Design review of the part built by this model. Coordinates are the model's own, in mm. Face numbers are marked on the shaded views. A direction names the side the tool comes from. Coordinates: 2 decimals unless noted, no trailing zeros. Loops run counter-clockwise (first coordinate to the right, second up) from the corner with the lowest first, then second, coordinate; pieces in that order, holes last.
Q1. Machinability: for the marked faces 1 and 2, which of the approach directions +Z, -Z, +X, -X, +Y, -Y give a long, thin tool a straight path to every point of the face, cutting with its end or side? Answer none if there is none.
Q2. For P1, Ø3, axis at x = 15, y = 4, coming from the -Z side; P2, Ø1, axis at x = -8.5, y = 2, coming from the +Z side; P3, Ø2, axis at x = 16, y = 3, coming from the -Z side, all flat-tipped, find the tip position at first contact; note any pin that passes through.
Q3. Add section C-C on y = 0.85. Give the boundary of the cut face in (x, z).
Q4. Add section D-D on x = 0. Give the boundary of the cut face in (y, z), and give its area (3 significant figures).
Q5. Add section A-A on x = -22. Give the boundary of the cut face in (y, z), and give its area (3 significant figures).
Q6. Draft analysis for pull direction X (two halves, no side actions). For the marked faces 3 and 4, state which applies: released by +X, released by -X, zero draft, split by the parting line, or undercut.
Q7. Add section B-B on z = -22. Give the boundary of the cut face in (x, y).
Q8. Wall thickness on probe 1 along X at (y, z) = (0.9, 1); probe 2 along X at (y, z) = (1.9, 22): over which ranges is each line inside the solid? List them lowest first.
```python
from build123d import *

# Parameters (mm, degrees)
SKETCH1_R           = 1.5
BOSS_EXTRUDE1_DEPTH = 3
BOSS_EXTRUDE2_START = 3
SKETCH1_4_R         = 1.5
SKETCH1_4_R_2       = 16
SKETCH1_4_R_3       = 13
BOSS_EXTRUDE2_DEPTH = 2


with BuildPart() as part:
    # Sketch1 → Boss-Extrude1 (new body)
    with BuildSketch(Plane(origin=(0, 0, 0), x_dir=(1, 0, 0), z_dir=(0, 1, 0))):
        with BuildLine():
            ThreePointArc((19.8125, 2.732186624), (14.142135624, 14.142135624), (2.732186624, 19.8125))
            ThreePointArc((2.732186624, 19.8125), (0, 25.5), (-2.732186624, 19.8125))
            ThreePointArc((-2.732186624, 19.8125), (-14.142135624, 14.142135624), (-19.8125, 2.732186624))
            ThreePointArc((-19.8125, 2.732186624), (-25.5, 0), (-19.8125, -2.732186624))
            ThreePointArc((-19.8125, -2.732186624), (-14.142135624, -14.142135624), (-2.732186624, -19.8125))
            ThreePointArc((-2.732186624, -19.8125), (0, -25.5), (2.732186624, -19.8125))
            ThreePointArc((2.732186624, -19.8125), (14.142135624, -14.142135624), (19.8125, -2.732186624))
            ThreePointArc((19.8125, -2.732186624), (25.5, 0), (19.8125, 2.732186624))
        make_face()
        with Locations((22, 0)):
            Circle(SKETCH1_R, mode=Mode.SUBTRACT)
        with Locations((0, 22)):
            Circle(SKETCH1_R, mode=Mode.SUBTRACT)
        with Locations((0, -22)):
            Circle(SKETCH1_R, mode=Mode.SUBTRACT)
        with Locations((-22, 0)):
            Circle(SKETCH1_R, mode=Mode.SUBTRACT)
    extrude(amount=BOSS_EXTRUDE1_DEPTH)

    # Sketch1_4 → Boss-Extrude2 (add)
    with BuildSketch(Plane(origin=(0, 0, 0), x_dir=(1, 0, 0), z_dir=(0, 1, 0)).offset(BOSS_EXTRUDE2_START)):
        with BuildLine():
            ThreePointArc((-2.732186624, -19.8125), (0, -25.5), (2.732186624, -19.8125))
            ThreePointArc((2.732186624, -19.8125), (0, -20), (-2.732186624, -19.8125))
        make_face()
        with Locations((0, -22)):
            Circle(SKETCH1_4_R, mode=Mode.SUBTRACT)
        with BuildLine():
            ThreePointArc((19.8125, 2.732186624), (19.953069939, 1.369306394), (20, 0))
            ThreePointArc((20, 0), (19.953069939, -1.369306394), (19.8125, -2.732186624))
            ThreePointArc((19.8125, -2.732186624), (25.5, 0), (19.8125, 2.732186624))
        make_face()
        with Locations((22, 0)):
            Circle(SKETCH1_4_R, mode=Mode.SUBTRACT)
        with BuildLine():
            ThreePointArc((-2.732186624, 19.8125), (0, 20), (2.732186624, 19.8125))
            ThreePointArc((2.732186624, 19.8125), (0, 25.5), (-2.732186624, 19.8125))
        make_face()
        with Locations((0, 22)):
            Circle(SKETCH1_4_R, mode=Mode.SUBTRACT)
        with BuildLine():
            ThreePointArc((-19.8125, -2.732186624), (-20, 0), (-19.8125, 2.732186624))
            ThreePointArc((-19.8125, 2.732186624), (-25.5, 0), (-19.8125, -2.732186624))
        make_face()
        with Locations((-22, 0)):
            Circle(SKETCH1_4_R, mode=Mode.SUBTRACT)
        Circle(SKETCH1_4_R_2)
        Circle(SKETCH1_4_R_3, mode=Mode.SUBTRACT)
    extrude(amount=BOSS_EXTRUDE2_DEPTH)


solid = part.part
```
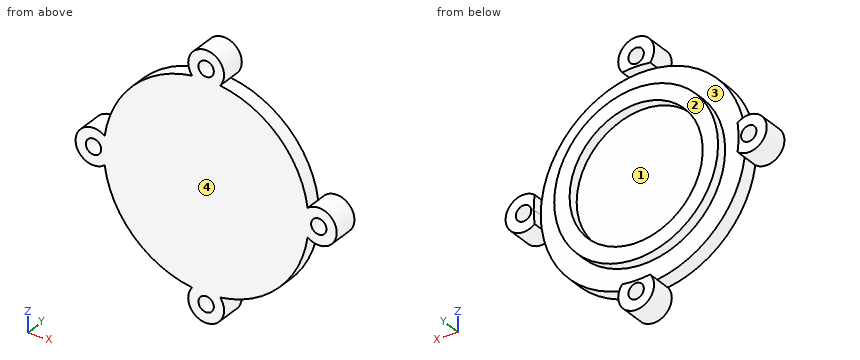
Entries:
1. face 1: +Y
1. face 2: +Z, -Z, +X, -X, +Y
2. P1: stops at z = -14.4
2. P2: stops at z = 18.33
2. P3: stops at z = -13.23
3. outline: (-19.81, -2.73) arc R20 ccw to (-2.73, -19.81) arc R3.5 ccw (long way) to (2.73, -19.81) arc R20 ccw to (19.81, -2.73) arc R3.5 ccw (long way) to (19.81, 2.73) arc R20 ccw to (2.73, 19.81) arc R3.5 ccw (long way) to (-2.73, 19.81) arc R20 ccw to (-19.81, 2.73) arc R3.5 ccw (long way) to start; hole circle Ø3 at (-22, 0); hole circle Ø3 at (0, -22); hole circle Ø3 at (0, 22); hole circle Ø3 at (22, 0)
4. outline: (0, -25.5) - (5, -25.5) - (5, -23.5) - (0, -23.5) - close; (0, -20.5) - (5, -20.5) - (5, -20) - (3, -20) - (3, -16) - (5, -16) - (5, -13) - (3, -13) - (3, 13) - (5, 13) - (5, 16) - (3, 16) - (3, 20) - (5, 20) - (5, 20.5) - (0, 20.5) - close; (0, 23.5) - (5, 23.5) - (5, 25.5) - (0, 25.5) - close
4. area: 157 mm2
5. outline: (0, -3.5) - (5, -3.5) - (5, -1.5) - (0, -1.5) - close; (0, 1.5) - (5, 1.5) - (5, 3.5) - (0, 3.5) - close
5. area: 20.0 mm2
6. face 3: undercut
6. face 4: zero draft
7. outline: (-3.5, 0) - (-1.5, 0) - (-1.5, 5) - (-3.5, 5) - close; (1.5, 0) - (3.5, 0) - (3.5, 5) - (1.5, 5) - close
8. probe 1: x = -25.35 to -23.12, -20.88 to 20.88, 23.12 to 25.35
8. probe 2: x = -3.5 to -1.5, 1.5 to 3.5
